Geometry check sheet. Reference: the model listing, model coordinates, mm. Face numbers are marked on the shaded views. Give positions to 0.01 mm unless a question says otherwise; leave off trailing zeros. Loops run counter-clockwise (first coordinate to the right, second up) from the corner with the lowest first, then second, coordinate; pieces in that order, holes last. Notation, with made-up numbers: (44.5, -25.75) - (49.5, -25.75) arc R24 cw to (49.5, 7.25) - close; hole circle Ø6 at (59, -28.75). An arc over 180 degrees is marked (long way). Write item = value, one per line. Start each with the question number.
from build123d import *

# Parameters (mm, degrees)
SKETCH1_W            = 80
SKETCH1_H            = 36
PCB_DEPTH            = 1.55
SKETCH2_R            = 1.55
MOUNTINGHOLES_DEPTH  = 44.890801998
SKETCH3_R            = 2.65
PADS_DEPTH           = 0.01
SKETCH4_R            = 0.5
CONNECTERHOLES_DEPTH = 44.890801998
SKETCH5_W            = 71
SKETCH5_H            = 24
PANELBODY_DEPTH      = 7.5
SKETCH6_W            = 64.5
SKETCH6_H            = 14.5
SCREEN_DEPTH         = 0.1


with BuildPart() as part:
    # Sketch1 → PCB (new body)
    with BuildSketch(Plane(origin=(0, 0, 0), x_dir=(1, 0, 0), z_dir=(0, 1, 0))):
        Rectangle(SKETCH1_W, SKETCH1_H)
    extrude(amount=PCB_DEPTH)

    # Sketch2 → MountingHoles (cut, through all)
    with BuildSketch(Plane(origin=(0, 1.55, 0), x_dir=(1, 0, 0), z_dir=(0, 1, 0))):
        with Locations(Location((-37.5, 15.575, 0), (0, 0, 270))):
            Circle(SKETCH2_R)
        with Locations(Location((37.5, 15.575, 0), (0, 0, 270))):
            Circle(SKETCH2_R)
        with Locations(Location((37.5, -15.575, 0), (0, 0, 270))):
            Circle(SKETCH2_R)
        with Locations(Location((-37.5, -15.575, 0), (0, 0, 270))):
            Circle(SKETCH2_R)
    extrude(amount=-MOUNTINGHOLES_DEPTH, mode=Mode.SUBTRACT)

    # Sketch3 → Pads (cut)
    with BuildSketch(Plane(origin=(0, 1.55, 0), x_dir=(1, 0, 0), z_dir=(0, 1, 0))):
        with Locations((-37.5, 15.575)):
            Circle(SKETCH3_R)
        with Locations((37.5, 15.575)):
            Circle(SKETCH3_R)
        with Locations((37.5, -15.575)):
            Circle(SKETCH3_R)
        with Locations((-37.5, -15.575)):
            Circle(SKETCH3_R)
        with BuildLine():
            Line((-32.9, 18), (-31.1, 18))
            Line((-31.1, 18), (-31.1, 16))
            ThreePointArc((-31.1, 16), (-32, 15.1), (-32.9, 16))
            Line((-32.9, 16), (-32.9, 18))
        make_face()
        with BuildLine():
            Line((-30.36, 18), (-30.36, 16))
            ThreePointArc((-30.36, 16), (-29.46, 15.1), (-28.56, 16))
            Line((-28.56, 16), (-28.56, 18))
            Line((-28.56, 18), (-30.36, 18))
        make_face()
        with BuildLine():
            Line((-27.82, 18), (-27.82, 16))
            ThreePointArc((-27.82, 16), (-26.92, 15.1), (-26.02, 16))
            Line((-26.02, 16), (-26.02, 18))
            Line((-26.02, 18), (-27.82, 18))
        make_face()
        with BuildLine():
            Line((-25.28, 18), (-25.28, 16))
            ThreePointArc((-25.28, 16), (-24.38, 15.1), (-23.48, 16))
            Line((-23.48, 16), (-23.48, 18))
            Line((-23.48, 18), (-25.28, 18))
        make_face()
        with BuildLine():
            Line((-22.74, 18), (-22.74, 16))
            ThreePointArc((-22.74, 16), (-21.84, 15.1), (-20.94, 16))
            Line((-20.94, 16), (-20.94, 18))
            Line((-20.94, 18), (-22.74, 18))
        make_face()
        with BuildLine():
            Line((-20.2, 18), (-20.2, 16))
            ThreePointArc((-20.2, 16), (-19.3, 15.1), (-18.4, 16))
            Line((-18.4, 16), (-18.4, 18))
            Line((-18.4, 18), (-20.2, 18))
        make_face()
        with BuildLine():
            Line((-17.66, 18), (-17.66, 16))
            ThreePointArc((-17.66, 16), (-16.76, 15.1), (-15.86, 16))
            Line((-15.86, 16), (-15.86, 18))
            Line((-15.86, 18), (-17.66, 18))
        make_face()
        with BuildLine():
            Line((-15.12, 18), (-15.12, 16))
            ThreePointArc((-15.12, 16), (-14.22, 15.1), (-13.32, 16))
            Line((-13.32, 16), (-13.32, 18))
            Line((-13.32, 18), (-15.12, 18))
        make_face()
        with BuildLine():
            Line((-12.58, 18), (-12.58, 16))
            ThreePointArc((-12.58, 16), (-11.68, 15.1), (-10.78, 16))
            Line((-10.78, 16), (-10.78, 18))
            Line((-10.78, 18), (-12.58, 18))
        make_face()
        with BuildLine():
            Line((-10.04, 18), (-10.04, 16))
            ThreePointArc((-10.04, 16), (-9.14, 15.1), (-8.24, 16))
            Line((-8.24, 16), (-8.24, 18))
            Line((-8.24, 18), (-10.04, 18))
        make_face()
        with BuildLine():
            Line((-7.5, 18), (-7.5, 16))
            ThreePointArc((-7.5, 16), (-6.6, 15.1), (-5.7, 16))
            Line((-5.7, 16), (-5.7, 18))
            Line((-5.7, 18), (-7.5, 18))
        make_face()
        with BuildLine():
            Line((-4.96, 18), (-4.96, 16))
            ThreePointArc((-4.96, 16), (-4.06, 15.1), (-3.16, 16))
            Line((-3.16, 16), (-3.16, 18))
            Line((-3.16, 18), (-4.96, 18))
        make_face()
        with BuildLine():
            Line((-2.42, 18), (-2.42, 16))
            ThreePointArc((-2.42, 16), (-1.52, 15.1), (-0.62, 16))
            Line((-0.62, 16), (-0.62, 18))
            Line((-0.62, 18), (-2.42, 18))
        make_face()
        with BuildLine():
            Line((0.12, 18), (0.12, 16))
            ThreePointArc((0.12, 16), (1.02, 15.1), (1.92, 16))
            Line((1.92, 16), (1.92, 18))
            Line((1.92, 18), (0.12, 18))
        make_face()
        with BuildLine():
            Line((2.66, 18), (2.66, 16))
            ThreePointArc((2.66, 16), (3.56, 15.1), (4.46, 16))
            Line((4.46, 16), (4.46, 18))
            Line((4.46, 18), (2.66, 18))
        make_face()
        with BuildLine():
            Line((5.2, 18), (5.2, 16))
            ThreePointArc((5.2, 16), (6.1, 15.1), (7, 16))
            Line((7, 16), (7, 18))
            Line((7, 18), (5.2, 18))
        make_face()
    extrude(amount=-PADS_DEPTH, mode=Mode.SUBTRACT)

    # Sketch4 → ConnecterHoles (cut, through all)
    with BuildSketch(Plane(origin=(0, 1.55, 0), x_dir=(1, 0, 0), z_dir=(0, 1, 0))):
        with Locations(Location((-32, 16, 0), (0, 0, 270))):
            Circle(SKETCH4_R)
        with Locations(Location((-29.46, 16, 0), (0, 0, 270))):
            Circle(SKETCH4_R)
        with Locations(Location((-26.92, 16, 0), (0, 0, 270))):
            Circle(SKETCH4_R)
        with Locations(Location((-24.38, 16, 0), (0, 0, 270))):
            Circle(SKETCH4_R)
        with Locations(Location((-21.84, 16, 0), (0, 0, 270))):
            Circle(SKETCH4_R)
        with Locations(Location((-19.3, 16, 0), (0, 0, 270))):
            Circle(SKETCH4_R)
        with Locations(Location((-16.76, 16, 0), (0, 0, 270))):
            Circle(SKETCH4_R)
        with Locations(Location((-14.22, 16, 0), (0, 0, 270))):
            Circle(SKETCH4_R)
        with Locations(Location((-11.68, 16, 0), (0, 0, 270))):
            Circle(SKETCH4_R)
        with Locations(Location((-9.14, 16, 0), (0, 0, 270))):
            Circle(SKETCH4_R)
        with Locations(Location((-6.6, 16, 0), (0, 0, 270))):
            Circle(SKETCH4_R)
        with Locations(Location((-4.06, 16, 0), (0, 0, 270))):
            Circle(SKETCH4_R)
        with Locations(Location((-1.52, 16, 0), (0, 0, 270))):
            Circle(SKETCH4_R)
        with Locations(Location((1.02, 16, 0), (0, 0, 270))):
            Circle(SKETCH4_R)
        with Locations(Location((3.56, 16, 0), (0, 0, 270))):
            Circle(SKETCH4_R)
        with Locations(Location((6.1, 16, 0), (0, 0, 270))):
            Circle(SKETCH4_R)
    extrude(amount=-CONNECTERHOLES_DEPTH, mode=Mode.SUBTRACT)

    # Sketch5 → PanelBody (add)
    with BuildSketch(Plane(origin=(0, 1.55, 0), x_dir=(1, 0, 0), z_dir=(0, 1, 0))):
        with Locations((0, -0.6)):
            Rectangle(SKETCH5_W, SKETCH5_H)
    extrude(amount=PANELBODY_DEPTH)

    # Sketch6 → Screen (cut)
    with BuildSketch(Plane(origin=(0, 9.05, 0), x_dir=(1, 0, 0), z_dir=(0, 1, 0))):
        with Locations((0, -0.6)):
            Rectangle(SKETCH6_W, SKETCH6_H)
    extrude(amount=-SCREEN_DEPTH, mode=Mode.SUBTRACT)


solid = part.part
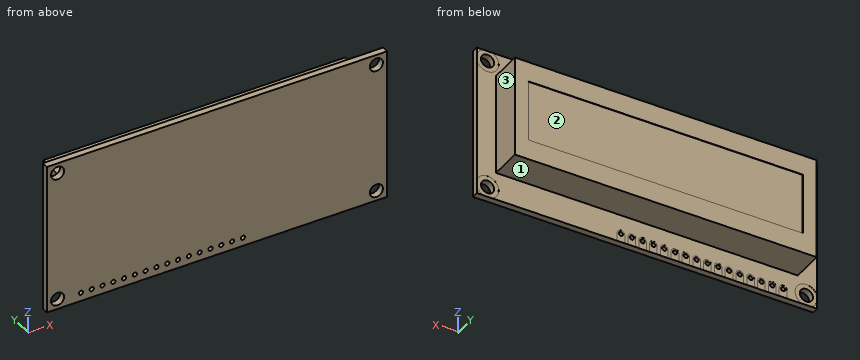
1) Cross-section at D-D on y = 3.5. Enter the section's corners in (x, z).
2) Cross-section at A-A on x = -37.5. Enter the section's corners in (y, z) (3 decimals).
3) Material ranges on line 1 along X through (y, z) = (7.25, 1); line 2 along Z through (x, y) = (16, 5.5); line 3 along Y through (x, z) = (25, -0.5), recorded low to high.
4) Release check for a two-part mould opening along X. For the marked faces 1, 2 and 3 record: pulls with the +X half, pulls with the -X half, needs draft (parallel to the pull), parting line crosses it, or undercut.
5) Cross-section at C-C on x = 8. Enter the section's corners in (y, z).
6) Gauge pin test, flat ends, axial feed: P1, Ø2, axis at x = -19, z = -16, coming from the +Y side; P2, Ø4, axis at y = 6.5, z = -7.5, coming from the -X side; P3, Ø4, axis at x = -10.5, z = 7.5, coming from the -Y side; P4, Ø4, axis at y = 7, z = -13.5, coming from the -X side. Record the tip position at first contact, or that the pin passes through.
7) Cross-section at B-B on z = -10. Enter the section's corners in (x, y).
Checked values:
q1.outline = (-35.5, -11.4) - (35.5, -11.4) - (35.5, 12.6) - (-35.5, 12.6) - close
q2.outline = (0, -18) - (1.54, -18) - (1.54, -17.125) - (0, -17.125) - close; (0, -14.025) - (1.54, -14.025) - (1.54, -12.925) - (1.55, -12.925) - (1.55, 12.925) - (1.54, 12.925) - (1.54, 14.025) - (0, 14.025) - close; (0, 17.125) - (1.54, 17.125) - (1.54, 18) - (0, 18) - close
q3.line_1 = -35.5 to 35.5
q3.line_2 = -11.4 to 12.6
q3.line_3 = 0 to 8.95
q4.face_1 = needs draft
q4.face_2 = undercut
q4.face_3 = pulls with the +X half
q5.outline = (0, -18) - (1.55, -18) - (1.55, -11.4) - (9.05, -11.4) - (9.05, -6.65) - (8.95, -6.65) - (8.95, 7.85) - (9.05, 7.85) - (9.05, 12.6) - (1.55, 12.6) - (1.55, 18) - (0, 18) - close
q6.P1 = 1.55
q6.P2 = -35.5
q6.P3 = 0
q6.P4 = through
q7.outline = (-40, 0) - (40, 0) - (40, 1.55) - (35.5, 1.55) - (35.5, 9.05) - (-35.5, 9.05) - (-35.5, 1.55) - (-40, 1.55) - close
